Geometry check sheet. Reference: the model listing, model coordinates, mm. Give positions to 0.01 mm unless a question says otherwise; leave off trailing zeros. Order: outer loops, then holes, each group sorted by start corner. A loop starts at its lowest first (then second) coordinate and runs counter-clockwise, first axis right, second up.
from build123d import *

# Parameters (mm, degrees)
SKETCH1_R           = 2
BOSS_EXTRUDE1_DEPTH = 42
SKETCH2_W           = 0.5
SKETCH2_H           = 0.2
SKETCH3_W           = 0.2
SKETCH3_H           = 0.15
CUT_EXTRUDE1_DEPTH  = 3


with BuildPart() as part:
    # Sketch1 → Boss-Extrude1 (new body)
    with BuildSketch(Plane(origin=(0, 0, 0), x_dir=(1, 0, 0), z_dir=(0, 1, 0))):
        with Locations(Location((0, 0, 0), (0, 0, 90))):
            Circle(SKETCH1_R)
    extrude(amount=BOSS_EXTRUDE1_DEPTH)

    # Sketch2 → Cut-Revolve1 (revolve, cut)
    with BuildSketch(Plane(origin=(0, 0, 0), x_dir=(0, 0, -1), z_dir=(1, 0, 0))):
        with Locations((1.75, 0.9)):
            Rectangle(SKETCH2_W, SKETCH2_H)
    revolve(axis=Axis((0, 3.062104398, 0), (0, -1, 0)), mode=Mode.SUBTRACT)

    # Sketch3 → Cut-Extrude1 (cut)
    with BuildSketch(Plane(origin=(0, 42, 0), x_dir=(1, 0, 0), z_dir=(0, 1, 0))):
        with Locations((0, 1.925)):
            Rectangle(SKETCH3_W, SKETCH3_H)
    extrude(amount=-CUT_EXTRUDE1_DEPTH, mode=Mode.SUBTRACT)


solid = part.part
Item 1: Sectioned sample at A-A (x = -0.9). Enter the section's corners in (y, z), and give its area (3 significant figures).
Reported:
outline: (0, -1.79) - (0.8, -1.79) - (0.8, -1.2) - (1, -1.2) - (1, -1.79) - (42, -1.79) - (42, 1.79) - (1, 1.79) - (1, 1.2) - (0.8, 1.2) - (0.8, 1.79) - (0, 1.79) - close
area: 150 mm2
Item 2: Scan lines: L1, parallel to Y at x = 0.9, z = 1.7; L2, parallel to X at y = 33, z = -0.15; L3, parallel to Z at x = 0, y = 40. Record each from-to range of solid material in increasing order.
Reported:
L1: y = 0 to 0.8, 1 to 42
L2: x = -1.99 to 1.99
L3: z = -1.85 to 2
Item 3: Sectioned sample at B-B (z = -0.9). Enter the section's corners in (x, y).
Reported:
outline: (-1.79, 0) - (1.79, 0) - (1.79, 0.8) - (1.2, 0.8) - (1.2, 1) - (1.79, 1) - (1.79, 42) - (-1.79, 42) - (-1.79, 1) - (-1.2, 1) - (-1.2, 0.8) - (-1.79, 0.8) - close
Item 4: Sectioned sample at C-C (y = 6). Enter the section's corners in (x, z).
Reported:
outline: circle Ø4 at (0, 0)
